Could you check a few things on this drawing? It's one solid part, dimensions in mm from its lowest x, y, z. Give positions to 0.01 mm unless a question says otherwise; leave off trailing zeros. Order: outer loops, then holes, each group sorted by start corner. A loop starts at its lowest first (then second) coordinate and runs counter-clockwise, first axis right, second up.
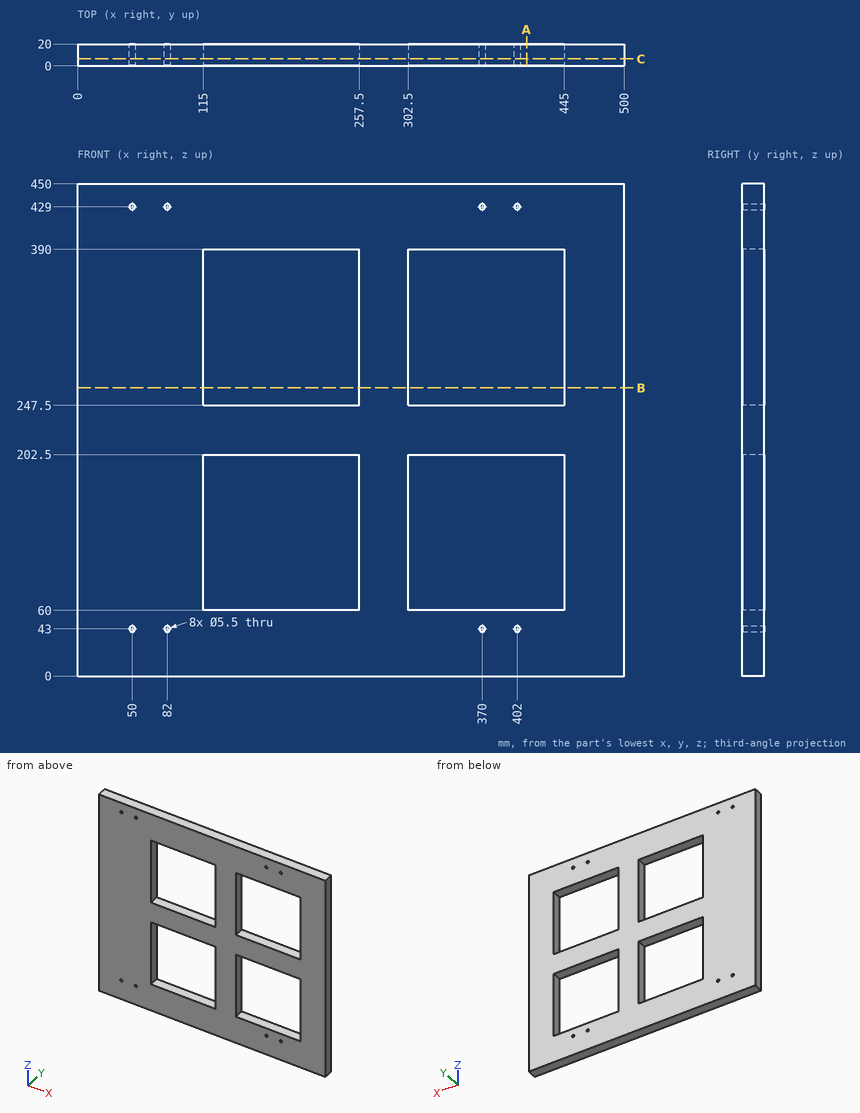
Item 1: Imagine slicing it at A-A on x = 410.5. List the corners of the cut face in (y, z) for me, then the cut area to 3 significant figures.
Findings:
outline: (0, 0) - (20, 0) - (20, 60) - (0, 60) - close; (0, 202.5) - (20, 202.5) - (20, 247.5) - (0, 247.5) - close; (0, 390) - (20, 390) - (20, 450) - (0, 450) - close
area: 3,300 mm2
Item 2: Imagine slicing it at B-B on z = 263.5. List the corners of the cut face in (x, y) for me.
Findings:
outline: (0, 0) - (115, 0) - (115, 20) - (0, 20) - close; (257.5, 0) - (302.5, 0) - (302.5, 20) - (257.5, 20) - close; (445, 0) - (500, 0) - (500, 20) - (445, 20) - close
Item 3: Imagine slicing it at C-C on y = 6.5. Give the number of separate pieces and of enclosed holes in the cut face, then the cut area to 3 significant figures.
Findings:
separate pieces: 1
enclosed holes: 12
area: 144,000 mm2
Item 4: For pin 1 (9 mm diameter, centred on x = 50, z = 43, fed in from -Y); pin 2 (3.5 mm diameter, centred on x = 50, z = 429, fed in from -Y), each with a flat end and sliding along its axis, tell me the tip position at first contact or that it passes through.
Findings:
pin 1: stops at y = 0
pin 2: passes through
Item 5: Please list where these lines run through material, in increasing order: line 1 along X through (y, z) = (11, 43); line 2 along Z through (x, y) = (223.5, 8.25); line 3 along X through (y, z) = (3.5, 300.5).
Findings:
line 1: x = 0 to 47.25, 52.75 to 79.25, 84.75 to 367.25, 372.75 to 399.25, 404.75 to 500
line 2: z = 0 to 60, 202.5 to 247.5, 390 to 450
line 3: x = 0 to 115, 257.5 to 302.5, 445 to 500
